from build123d import *

# Parameters (mm, degrees)
SKETCH1_R           = 2.125
SKETCH1_R_2         = 3
SKETCH1_W           = 6.35
SKETCH1_H           = 6
SKETCH1_W_2         = 12.7
SKETCH1_H_2         = 5.9944
BOSS_EXTRUDE1_DEPTH = 5.9944


with BuildPart() as part:
    # Sketch1 → Boss-Extrude1 (new body)
    with BuildSketch(Plane(origin=(0, 0, 0), x_dir=(-1, 0, 0), z_dir=(0, 0, 1))):
        with BuildLine():
            Line((72.098749996, 7.383354962), (72.098749996, -6.840645038))
            Line((72.098749996, -6.840645038), (65.748749996, -6.840645038))
            Line((65.748749996, -6.840645038), (65.748749996, -12.840645038))
            Line((65.748749996, -12.840645038), (72.098749996, -12.840645038))
            Line((72.098749996, -12.840645038), (72.098749996, -42.840645038))
            Line((72.098749996, -42.840645038), (72.098749996, -47.734229729))
            ThreePointArc((72.098749996, -47.734229729), (69.866903669, -53.122383402), (64.478749996, -55.354229729))
            Line((64.478749996, -55.354229729), (51.652589936, -55.354229729))
            Line((51.652589936, -55.354229729), (45.302589935, -55.354229729))
            Line((45.302589935, -55.354229729), (26.252589932, -55.354229729))
            Line((26.252589932, -55.354229729), (-35.770420068, -55.354229729))
            ThreePointArc((-35.770420068, -55.354229729), (-40.260548128, -53.494357789), (-42.120420068, -49.004229729))
            Line((-42.120420068, -49.004229729), (-42.120420068, 42.61894002))
            ThreePointArc((-42.120420068, 42.61894002), (-34.68093231, 60.579452262), (-16.720420068, 68.01894002))
            Line((-16.720420068, 68.01894002), (56.858749996, 68.01894002))
            ThreePointArc((56.858749996, 68.01894002), (67.635057342, 63.555247365), (72.098749996, 52.77894002))
            Line((72.098749996, 52.77894002), (72.098749996, 13.383354962))
            Line((72.098749996, 13.383354962), (65.748749996, 13.383354962))
            Line((65.748749996, 13.383354962), (65.748749996, 7.383354962))
            Line((65.748749996, 7.383354962), (72.098749996, 7.383354962))
        make_face()
        with Locations((-10.170420063, -18.840645038)):
            Circle(SKETCH1_R, mode=Mode.SUBTRACT)
        with Locations((13.829579937, -18.840645038)):
            Circle(SKETCH1_R, mode=Mode.SUBTRACT)
        with Locations((13.829579937, -36.840645038)):
            Circle(SKETCH1_R, mode=Mode.SUBTRACT)
        with Locations((-10.170420063, -36.840645038)):
            Circle(SKETCH1_R, mode=Mode.SUBTRACT)
        with Locations((-28.770420063, -43.34064498)):
            Circle(SKETCH1_R_2, mode=Mode.SUBTRACT)
        with Locations((-28.770420063, -12.34064498)):
            Circle(SKETCH1_R_2, mode=Mode.SUBTRACT)
        with Locations((42.848749997, -18.840645038)):
            Circle(SKETCH1_R, mode=Mode.SUBTRACT)
        with Locations((66.848749997, -18.840645038)):
            Circle(SKETCH1_R, mode=Mode.SUBTRACT)
        with Locations((-28.770420063, 9.67852502)):
            Circle(SKETCH1_R_2, mode=Mode.SUBTRACT)
        with Locations((-28.770420063, 40.67852502)):
            Circle(SKETCH1_R_2, mode=Mode.SUBTRACT)
        with Locations((66.848749997, -36.840645038)):
            Circle(SKETCH1_R, mode=Mode.SUBTRACT)
        with Locations((42.848749997, -36.840645038)):
            Circle(SKETCH1_R, mode=Mode.SUBTRACT)
        with Locations((-10.170420063, 34.178525078)):
            Circle(SKETCH1_R, mode=Mode.SUBTRACT)
        with Locations((13.829579937, 34.178525078)):
            Circle(SKETCH1_R, mode=Mode.SUBTRACT)
        with Locations((-10.170420063, 16.178525078)):
            Circle(SKETCH1_R, mode=Mode.SUBTRACT)
        with Locations((13.829579937, 16.178525078)):
            Circle(SKETCH1_R, mode=Mode.SUBTRACT)
        with Locations((49.873749996, 10.383354962)):
            Rectangle(SKETCH1_W, SKETCH1_H, mode=Mode.SUBTRACT)
        with BuildLine():
            Line((34.198749996, 55.383354962), (34.198749996, 25.383354962))
            ThreePointArc((34.198749996, 25.383354962), (32.098749996, 23.283354962), (29.998749996, 25.383354962))
            Line((29.998749996, 25.383354962), (29.998749996, 55.383354962))
            ThreePointArc((29.998749996, 55.383354962), (32.098749996, 57.483354962), (34.198749996, 55.383354962))
        make_face(mode=Mode.SUBTRACT)
        with BuildLine():
            Line((64.198749996, 55.383354962), (64.198749996, 25.383354962))
            ThreePointArc((64.198749996, 25.383354962), (62.098749996, 23.283354962), (59.998749996, 25.383354962))
            Line((59.998749996, 25.383354962), (59.998749996, 55.383354962))
            ThreePointArc((59.998749996, 55.383354962), (62.098749996, 57.483354962), (64.198749996, 55.383354962))
        make_face(mode=Mode.SUBTRACT)
        with Locations((49.873749996, -9.840645038)):
            Rectangle(SKETCH1_W, SKETCH1_H, mode=Mode.SUBTRACT)
        with Locations((-29.420420063, -1.33105998)):
            Rectangle(SKETCH1_W_2, SKETCH1_H_2, mode=Mode.SUBTRACT)
        with Locations((-4.020420063, -1.33105998)):
            Rectangle(SKETCH1_W_2, SKETCH1_H_2, mode=Mode.SUBTRACT)
        with Locations((21.379579937, -1.33105998)):
            Rectangle(SKETCH1_W_2, SKETCH1_H_2, mode=Mode.SUBTRACT)
        with Locations((46.779579937, -1.33105998)):
            Rectangle(SKETCH1_W_2, SKETCH1_H_2, mode=Mode.SUBTRACT)
    extrude(amount=BOSS_EXTRUDE1_DEPTH)


solid = part.part
Model file for the job. Use its own axes, mm. A direction names the side the tool comes from. Round coordinates to 2 decimals unless told otherwise and drop trailing zeros. Order: outer loops, then holes, each group sorted by start corner. A loop starts at its lowest first (then second) coordinate and runs counter-clockwise, first axis right, second up.
(1) Band-saw the part on C-C (z = 3.05). Give the number of separate pieces and of enclosed holes in the cut face, then the cut area to 3 significant figures.
(2) Drill centre lines: line 1 (X direction, y = -26.5, z = 4.25); line 2 (X direction, y = 2, z = 0.5); line 3 (Y direction, x = -2, z = 4.55). Where is each one in solid material? Low to high.
(3) Band-saw the part on B-B (x = 34). List the corners of the cut face in (y, z).
(4) Pin check, flat tips, straight feed: pin 1 (1.8 mm diameter, centred on x = 27.5, z = 4, fed in from -Y); pin 2 (5 mm diameter, centred on x = -66.85, y = 36.84, fed in from -Z); pin 3 (3 mm diameter, centred on x = 24, z = 1, fed in from -Y). Stop position of each tip, or through.
(5) Pull direction X, two halves, no side cores. Call faces 1 (the face through (-20, -68.019, 3)), 2 (the face through (-72.099, 0, 3)), 3 (the face through (-50, 12.841, 3)): released by +X, released by -X, zero draft, split by the parting line, or undercut.
(6) Band-saw the part on A-A (y = -49). List the corners of the cut face in (x, z).
(7) 3-axis set-ups, long thin cutter, end or side, ignore diameter. For faces 4 (the face through (42.12, 4, 3)), 5 (the face through (4, 4.328, 3)): which of +Z, -Z, +X, -X, +Y, -Y reach the whole face in a straight line?
Verdict:
1. separate pieces: 1
1. enclosed holes: 24
1. area: 12,900 mm2
2. line 1: x = -72.1 to -64.2, -60 to -34.2, -30 to 42.12
2. line 2: x = -72.1 to -53.13, -40.43 to -27.73, -15.03 to -2.33, 10.37 to 23.07, 35.77 to 42.12
2. line 3: y = -68.02 to -1.67, 4.33 to 55.35
3. outline: (-61.24, 0) - (-1.67, 0) - (-1.67, 5.99) - (-61.24, 5.99) - close; (4.33, 0) - (55.35, 0) - (55.35, 5.99) - (4.33, 5.99) - close
4. pin 1: stops at y = -66.02
4. pin 2: stops at z = 0
4. pin 3: stops at y = -67.35
5. face 1: zero draft
5. face 2: released by -X
5. face 3: undercut
6. outline: (-72.1, 0) - (-64.2, 0) - (-64.2, 5.99) - (-72.1, 5.99) - close; (-60, 0) - (-34.2, 0) - (-34.2, 5.99) - (-60, 5.99) - close; (-30, 0) - (41.31, 0) - (41.31, 5.99) - (-30, 5.99) - close
7. face 4: +Z, -Z, +X, +Y, -Y
7. face 5: +Z, -Z
